Solid Edge part; units mm, degrees
sketch "Sketch1" plane through (0, 0, 0) normal (0, -1, 0) x (1, 0, 0)
  line L0 (5, 5) -> (-5, 5)
  line L1 (-5, 5) -> (-5, -5)
  line L2 (-5, -5) -> (5, -5)
  line L3 (5, -5) -> (5, 5)
extrude "Protrusion1" add sketch "Sketch1" against normal blind 70
hole "Hole_1" at (0, 0, 0) direction (0, 1, 0) diameter 3.242 depth 25 thread major 4 thread length 2
Here's how the part is built. I have some questions about the finished solid (model axes, mm). A direction names the side the tool comes from. Coordinates: 2 decimals unless noted, no trailing zeros. Order: outer loops, then holes, each group sorted by start corner. A loop starts at its lowest first (then second) coordinate and runs counter-clockwise, first axis right, second up.
1) Imagine slicing it at B-B on z = 0. List the corners of the cut face in (x, y) for me, and give its area (3 significant figures).
2) Will this pin go through, and if not, where does the flat tip stop? pin 1 (2.5 mm diameter, centred on x = 0.5, z = 0, fed in from -Y).
3) We'd pull the mould along X, two halves only. Please class faces 1 (the face through (1.438, 12.675, -0.748)), 2 (the face through (-5, 35, 0)), 3 (the face through (0, 35, -5)): +X half, -X half, draft (parallel to the pull), parting line (faces both ways), or undercut.
4) Which directions (+Z, -Z, +X, -X, +Y, -Y) give clear straight access to the entire face, cutting with the end or side of a thin tool? Please do faces 4 (the face through (5, 35, 0)), 5 (the face through (0, 25, 0)).
5) Imagine slicing it at A-A on x = 0. List the corners of the cut face in (y, z) for me, and give its area (3 significant figures).
6) I need wall thicknesses on line 1 (X direction, y = 16.75, z = 0); line 2 (X direction, y = 7, z = 1). Which ranges of each line are inside material? Lowest first, please.
Response values:
1. outline: (-5, 0) - (-1.62, 0) - (-1.62, 25) - (1.62, 25) - (1.62, 0) - (5, 0) - (5, 70) - (-5, 70) - close
1. area: 619 mm2
2. pin 1: stops at y = 0
3. face 1: undercut
3. face 2: -X half
3. face 3: draft
4. face 4: +Z, -Z, +X, +Y, -Y
4. face 5: -Y
5. outline: (0, -5) - (70, -5) - (70, 5) - (0, 5) - (0, 1.62) - (25, 1.62) - (25, -1.62) - (0, -1.62) - close
5. area: 619 mm2
6. line 1: x = -5 to -1.62, 1.62 to 5
6. line 2: x = -5 to -1.28, 1.28 to 5
